Check sheet for the modelled part. Datum: model origin and axes. Units: mm. A direction names the side the tool comes from. Coordinates: 2 decimals unless noted, no trailing zeros. Loops run counter-clockwise (first coordinate to the right, second up) from the corner with the lowest first, then second, coordinate; pieces in that order, holes last.
```python
from build123d import *

# Parameters (mm, degrees)
F0_R     = 25
F1_DEPTH = 21
F2_R     = 21.75
F3_DEPTH = 6
F4_R     = 5
F5_DEPTH = 10
F6_SIZE  = 0.5
F7_R     = 4


with BuildPart() as f1:
    # F0 (on Top) → F1 (new body)
    with BuildSketch(Plane.XY):
        Circle(F0_R)
    extrude(amount=F1_DEPTH)

    # F2 (on face) → F3 (join)
    with BuildSketch(Plane.XY.offset(21)):
        Circle(F2_R)
    extrude(amount=F3_DEPTH)

    # F4 (on face) → F5 (cut)
    with BuildSketch(Plane.XY.offset(27)):
        Circle(F4_R)
    extrude(amount=-F5_DEPTH, mode=Mode.SUBTRACT)

    # F6
    f6_edges = [f1.edges().sort_by_distance(p)[0] for p in [
        (-21.75, 0, 27),
        (-25, 0, 21),
    ]]
    chamfer(f6_edges, length=F6_SIZE)

    # F7
    f7_edges = [f1.edges().sort_by_distance(p)[0] for p in [
        (-25, 0, 0),
    ]]
    fillet(f7_edges, radius=F7_R)


solid = f1.part
```
1) Section check C-C on z = 16.25. Enter the section's corners in (x, y).
Answer sheet:
outline: circle Ø50 at (0, 0)
2) Section check A-A on x = 0. Enter the section's corners in (y, z), plus the area to 3 significant figures.
Answer sheet:
outline: (-25, 4) arc R4 ccw to (-21, 0) - (21, 0) arc R4 ccw to (25, 4) - (25, 20.5) - (24.5, 21) - (21.75, 21) - (21.75, 26.5) - (21.25, 27) - (5, 27) - (5, 17) - (-5, 17) - (-5, 27) - (-21.25, 27) - (-21.75, 26.5) - (-21.75, 21) - (-24.5, 21) - (-25, 20.5) - close
area: 1,200 mm2
3) Mould release check, pull along X, two halves, no side actions. Record for faces 3 (the cylindrical face through (23.846, 7.509, 12.134)), 4 (the cylindrical face through (-1.08, -4.88, 22.07)), 5 (the flat face through (0, 0, 17)), 6 (the flat face through (0, 0, 0)): +X half, -X half, draft (parallel to the pull), parting line (faces both ways), or undercut.
Answer sheet:
face 3: parting line
face 4: undercut
face 5: undercut
face 6: draft
4) Set-up check for faces 1 (the flat face through (0, 22, 21)), 2 (the flat face through (4, -4, 27)): record each of +Z, -Z, +X, -X, +Y, -Y from which the full face is reachable in a straight line by a thin tool's end or side.
Answer sheet:
face 1: +Z
face 2: +Z, +X, -X, +Y, -Y
5) Scan lines: line 1 (Y direction, x = 0, z = 20.5); line 2 (Y direction, x = 0, z = 23); line 3 (X direction, y = -3.5, z = 18.25). Record each from-to range of solid material in increasing order.
Answer sheet:
line 1: y = -25 to -5, 5 to 25
line 2: y = -21.75 to -5, 5 to 21.75
line 3: x = -24.75 to -3.57, 3.57 to 24.75
6) Depth check by flat-ended pin: pin 1 (4 mm diameter, centred on x = -16, y = -18, fed in from +Z); pin 2 (6 mm diameter, centred on x = 0, y = 0, fed in from +Z); pin 3 (2 mm diameter, centred on x = -14, z = 17.5, fed in from -Y). Enter the tip coordinate at first touch or a pass-through.
Answer sheet:
pin 1: stops at z = 21
pin 2: stops at z = 17
pin 3: stops at y = -21.35
